Input: part model. Units: mm. Frame: model coordinates. Give positions to 0.01 mm unless a question says otherwise; leave off trailing zeros. Write each loop counter-clockwise with the first axis right and the second up, starting at its lowest first coordinate (ties: lowest second). Pieces come first, ordered by that corner, then holes. Notation, with made-up numbers: (-3.75, 59.25) - (38.25, 59.25) arc R27 ccw to (38.25, 80.25) - close; hole circle Ø6 at (6, 64). An arc over 180 degrees is marked (long way). Answer as a JSON object with one key per item and string values. Group by question number.
from build123d import *

# Parameters (mm, degrees)
F2_R     = 4.0386
F3_DEPTH = 3.4925
F4_DEPTH = 8.001


with BuildPart() as f1:
    # F0 (on Right) → F1 (revolve)
    with BuildSketch(Plane.YZ):
        Polygon((-1.907612, 10.818606), (0, 0), (4.445, 0), (2.537388, 10.818606), align=None)
    revolve(axis=Axis((0, 0.105105, 0), (0, 1, 0)))

    # F2 (on Front) → F3 (join)
    with BuildSketch(Plane.XZ):
        Circle(F2_R)
    extrude(amount=-F3_DEPTH)

    # F2 (on Front) → F4 (join)
    with BuildSketch(Plane.XZ):
        Circle(F2_R)
    extrude(amount=-F4_DEPTH)


solid = f1.part
1) Mould query, pull axis X, two halves, no side actions, for faces 1 (the face through (0, 8.001, 0)), 2 (the face through (0, 0, 0)), 3 (the face through (-10.56, 0.28, -2.35)). Classes: +X half, -X half, draft (parallel to the pull), parting line (faces both ways), or undercut.
2) Cut plane B-B on y = 1. Return the cut outline in (x, z), and give its area (3 significant figures).
3) Line query: line 1 along X through (y, z) = (1.75, 0); line 2 along X through (y, z) = (5, 0.5); line 3 along Z through (x, y) = (-4.5, 2.5). Output: solid intervals per line, ascending. Write a range as from..to.
4) Pin query (flat end, axial travel): P1, Ø3, axis at x = 1.5, y = 3, coming from the -Z side; P2, Ø3, axis at x = 0.5, z = 5.5, coming from the -Y side; P3, Ø5, axis at x = -6.5, z = 3, coming from the -Y side; P4, Ø4, axis at x = 2.5, z = -8, coming from the +Y side. Return the tip coordinate at first contact, or that it passes through.
5) Cut plane A-A on y = 4.5. Return the cut outline in (x, z), and give its area (3 significant figures).
Filled in:
{
 "1": {"face 1": "draft", "face 2": "undercut", "face 3": "parting line"},
 "2": {"outline": "circle Ø21.64 at (0, 0)", "area": "368 mm²"},
 "3": {"line 1": "x = -10.82..10.82", "line 2": "x = -4.01..4.01", "line 3": "z = -9.84..9.84"},
 "4": {"P1": "stops at z = -10.82", "P2": "stops at y = -1.24", "P3": "stops at y = -1.7", "P4": "stops at y = 3.32"},
 "5": {"outline": "circle Ø8.08 at (0, 0)", "area": "51.2 mm²"}
}
